Read the model definition and answer for the solid it produces. Units are mm, in the model's axes. A direction names the side the tool comes from. Coordinates: 2 decimals unless noted, no trailing zeros. One line per item, written item: value. Start each with the question number.
from build123d import *

# Parameters (mm, degrees)
CUT_EXTRUDE1_DEPTH      = 617.614952787
CUT_EXTRUDE1_DEPTH_BACK = 617.614952787
SKETCH2_R               = 8
CUT_EXTRUDE2_DEPTH      = 618.636624562
CUT_EXTRUDE2_DEPTH_BACK = 20
SKETCH3_R               = 8
SKETCH4_R               = 8
CUT_EXTRUDE3_DEPTH      = 15


with BuildPart() as part:
    # Sketch1 → Revolve1 (revolve)
    with BuildSketch(Plane.XY, mode=Mode.PRIVATE) as revolve1_sk:
        with BuildLine():
            Line((-365, 0), (-385, 0))
            Line((-385, 0), (-385, 13))
            Line((-385, 13), (-435, 13))
            Line((-435, 13), (-435, 20))
            ThreePointArc((-435, 20), (-432.071067812, 27.071067812), (-425, 30))
            Line((-425, 30), (-105, 30))
            ThreePointArc((-105, 30), (-90.857864376, 35.857864376), (-85, 50))
            Line((-85, 50), (-85, 55))
            Line((-85, 55), (-45, 55))
            Line((-45, 55), (-45, 15))
            Line((-45, 15), (-355, 15))
            ThreePointArc((-355, 15), (-362.071067812, 12.071067812), (-365, 5))
            Line((-365, 5), (-365, 0))
        make_face()
    revolve(revolve1_sk.sketch.rotate(Axis((0, 0, 0), (0, 1, 0)), 270), axis=Axis((0, 0, 0), (0, 1, 0)))

    # Sketch2 → Cut-Extrude1 (cut, two sides: drawn at the far end of the back side and taken through both)
    with BuildSketch(Plane.XZ.offset(-13).offset(-CUT_EXTRUDE1_DEPTH_BACK)):
        with Locations(Location((410, 0, 0), (0, 0, 270))):
            Circle(SKETCH2_R)
        with Locations(Location((289.913780286, -289.913780286, 0), (0, 0, 270))):
            Circle(SKETCH2_R)
        with Locations(Location((0, -410, 0), (0, 0, 270))):
            Circle(SKETCH2_R)
        with Locations(Location((-289.913780286, -289.913780286, 0), (0, 0, 270))):
            Circle(SKETCH2_R)
        with Locations(Location((-410, 0, 0), (0, 0, 270))):
            Circle(SKETCH2_R)
        with Locations(Location((-289.913780286, 289.913780286, 0), (0, 0, 270))):
            Circle(SKETCH2_R)
        with Locations(Location((0, 410, 0), (0, 0, 270))):
            Circle(SKETCH2_R)
        with Locations(Location((289.913780286, 289.913780286, 0), (0, 0, 270))):
            Circle(SKETCH2_R)
    extrude(amount=CUT_EXTRUDE1_DEPTH + CUT_EXTRUDE1_DEPTH_BACK, mode=Mode.SUBTRACT)

    # Sketch3 → Cut-Extrude2 (cut, two sides: drawn at the far end of the back side and taken through both)
    with BuildSketch(Plane(origin=(0, 55, 0), x_dir=(1, 0, 0), z_dir=(0, 1, 0)).offset(-CUT_EXTRUDE2_DEPTH_BACK)):
        with Locations(Location((70, 0, 0), (0, 0, 90))):
            Circle(SKETCH3_R)
        with Locations(Location((35, -60.621778265, 0), (0, 0, 90))):
            Circle(SKETCH3_R)
        with Locations(Location((-35, -60.621778265, 0), (0, 0, 90))):
            Circle(SKETCH3_R)
        with Locations(Location((-70, 0, 0), (0, 0, 90))):
            Circle(SKETCH3_R)
        with Locations(Location((-35, 60.621778265, 0), (0, 0, 90))):
            Circle(SKETCH3_R)
        with Locations(Location((35, 60.621778265, 0), (0, 0, 90))):
            Circle(SKETCH3_R)
    extrude(amount=CUT_EXTRUDE2_DEPTH + CUT_EXTRUDE2_DEPTH_BACK, mode=Mode.SUBTRACT)

    # Sketch4 → Cut-Extrude3 (cut)
    with BuildSketch(Plane(origin=(0, 30, 0), x_dir=(1, 0, 0), z_dir=(0, 1, 0))):
        with Locations(Location((-200, 0, 0), (0, 0, 270))):
            Circle(SKETCH4_R)
    extrude(amount=-CUT_EXTRUDE3_DEPTH, mode=Mode.SUBTRACT)


solid = part.part
1) Flat-ended cylindrical pins translate along their axes: P1, Ø13, axis at x = -70.5, z = -1, coming from the +Y side; P2, Ø18.5, axis at x = -289.91, z = 289.91, coming from the -Y side; P3, Ø4, axis at x = 161.5, z = -210.5, coming from the +Y side; P4, Ø17.5, axis at x = 72.5, z = 1, coming from the +Y side. Find the tip coordinate at first contact, or state that the pin passes through.
2) Determine the mould class of faces 4 (the flat face through (385, 13, -34)), 5 (the cylindrical face through (356.32, 2.46, 79.12)), 6 (the cylindrical face through (51.721, 52.535, 67.453)) for opening direction X: released by +X, released by -X, zero draft, split by the parting line, or undercut.
3) For faces 1 (the flat face through (74, 15, -5)), 2 (the flat face through (88, 30, -88)), 3 (the flat face through (37, 55, -37)), determine the directions among +Z, -Z, +X, -X, +Y, -Y from which every point of the face is accessible in a straight line to the end or side of a thin tool.
4) Straight lines are drawn through the part: L1, parallel to X at y = 12, z = 259; L2, parallel to Z at x = 310, y = 7.5; L3, parallel to X at y = 45, z = 0. For each, find the intervals that lie inside material, in ascending order.
Answer below:
1. P1: y = 35
1. P2: y = 13
1. P3: y = 30
1. P4: y = 55
2. face 4: zero draft
2. face 5: undercut
2. face 6: split by the parting line
3. face 1: -Y
3. face 2: +Y
3. face 3: +Z, -Z, +X, -X, +Y
4. L1: -284.86 to -253.11, 253.11 to 284.86
4. L2: -228.31 to -192.08, 192.08 to 228.31
4. L3: -85.64 to -78, -62 to -45, 45 to 62, 78 to 85.64
